from build123d import *

# Parameters (mm, degrees)
SKETCH1_W           = 16.764
SKETCH1_H           = 8.128
BOSS_EXTRUDE1_DEPTH = 35.814
BOSS_EXTRUDE2_DEPTH = 2.54


with BuildPart() as part:
    # Sketch1 → Boss-Extrude1 (new body)
    with BuildSketch(Plane(origin=(0, 0, 0), x_dir=(0, 0, -1), z_dir=(1, 0, 0))):
        with Locations((8.382, 4.064)):
            Rectangle(SKETCH1_W, SKETCH1_H)
    extrude(amount=BOSS_EXTRUDE1_DEPTH)

    # Sketch2 → Boss-Extrude2 (add)
    with BuildSketch(Plane.XY):
        with BuildLine():
            Line((1.27, 4.736473545), (1.27, 3.391526455))
            ThreePointArc((1.27, 3.391526455), (0.635, 2.756526455), (0, 3.391526455))
            Line((0, 3.391526455), (0, 4.736473545))
            ThreePointArc((0, 4.736473545), (0.635, 5.371473545), (1.27, 4.736473545))
        make_face()
    extrude(amount=BOSS_EXTRUDE2_DEPTH)


solid = part.part
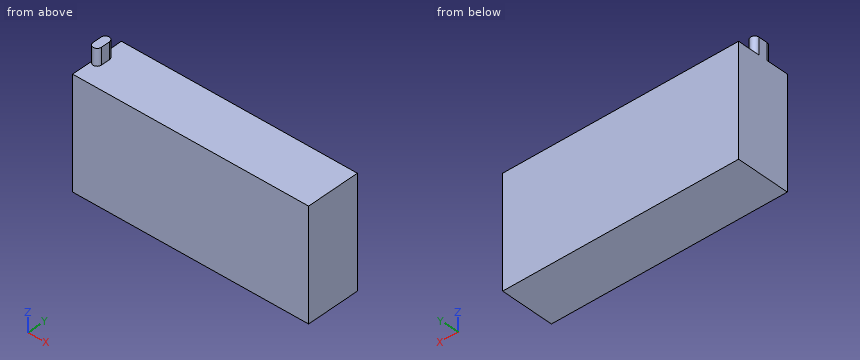
For this review, take the finished solid that the model builds, in its own axes (mm). Coordinates: 2 decimals unless noted, no trailing zeros. Loops run counter-clockwise (first coordinate to the right, second up) from the corner with the lowest first, then second, coordinate; pieces in that order, holes last. Notation, with made-up numbers: (61.5, 29) - (71.5, 29) arc R22 ccw to (71.5, 64) - close; hole circle Ø10 at (61.25, 33). An arc over 180 degrees is marked (long way). Use a Markdown table: item, result. Add a question column.
Item 1: For line 1 (Z direction, x = 18, y = 2.75), list the stretches that pass through material, from the lowest coordinate up.
Item 2: Insertion check: pin 1 Ø3 at (x, y) = (20, 5.5) entering from +Z. The pin has a flat end and moves straight along its axis. Give the tip position at first contact, or say it passes through.
Item 3: We need section A-A (x = 14.5). Give the boundary of the cut face in (y, z), and give its area (3 significant figures).
Item 4: We need section B-B (y = 7.25). Give the boundary of the cut face in (x, z), and give its area (3 significant figures).
Results list:
| question | item | result |
|---|---|---|
| 1 | line 1 | z = -16.76 to 0 |
| 2 | pin 1 | stops at z = 0 |
| 3 | outline | (0, -16.76) - (8.13, -16.76) - (8.13, 0) - (0, 0) - close |
| 3 | area | 136 mm^2 |
| 4 | outline | (0, -16.76) - (35.81, -16.76) - (35.81, 0) - (0, 0) - close |
| 4 | area | 600 mm^2 |
